Design review of the part built by this model. Coordinates are the model's own, in mm. A direction names the side the tool comes from. Coordinates: 2 decimals unless noted, no trailing zeros. Loops run counter-clockwise (first coordinate to the right, second up) from the corner with the lowest first, then second, coordinate; pieces in that order, holes last. Notation, with made-up numbers: M 27.25,-6 L 49.25,-6 A22 ccw 49.25,21 Z; hole C 76,1 d5. An arc over 180 degrees is marked long. Put each result on its own line as item: value. Start each with the question number.
(1) Clearance check with flat-ended pins moving along their axes: pin 1 (2 mm diameter, centred on y = 7, z = 7.5, fed in from -X); pin 2 (3.5 mm diameter, centred on x = 0, y = 9, fed in from -Z); pin 3 (3 mm diameter, centred on y = -2.5, z = 3.5, fed in from -X). State where each tip first meets the part, or that it passes through.
(2) Take a section at B-B, the plane x = 0. Count the separate pieces of the cut face and the enclosed holes in it, then the cut area to 4 significant figures.
(3) For faces 5 (the cylindrical face through (3.461, 9.056, 6.654)), 6 (the cylindrical face through (-7.493, -6.972, -0.33)), 7 (the conical face through (9.09, 0.17, -1.19)), list the 3-axis set-ups (+Z, -Z, +X, -X, +Y, -Y) from which the entire face can be reached by the end or side of a thin tool; tool diameter is ignored.
(4) Take a section at C-C, the plane y = 9. Give the boundary of the cut face in (x, z), then the cut area to 3 significant figures.
(5) Take a section at D-D, the plane y = -7.25. Give the boundary of the cut face in (x, z).
(6) The part is to be moulded in two halves that separate along X. For faces 1 (the cylindrical face through (11.547, 4.26, 4.788)), 2 (the cylindrical face through (-1.5, 9.07, 5.58)), 3 (the flat face through (0, 5, 8)), 4 (the cylindrical face through (-1.5, 9.07, -5.58)), say which applies: +X half, -X half, draft (parallel to the pull), parting line (faces both ways), or undercut.
(7) For probe 1 along X at (y, z) = (6.75, 0); probe 2 along Y at (x, z) = (0, -4.85); probe 3 along Y at (x, z) = (-6, 9.5), list the stretches that pass through material, from the lowest coordinate up. Write a range as [from, to].
(8) Take a section at A-A, the plane z = 0. Give the boundary of the cut face in (x, y).
```python
from build123d import *

# Parameters (mm, degrees)
SKETCH1_R                = 7.5
SKETCH1_R_2              = 4
BOSS_EXTRUDE1_DEPTH      = 13
BOSS_EXTRUDE1_DEPTH_BACK = 9
SKETCH1_4_R              = 12.5
SKETCH1_4_R_2            = 7.5
BOSS_EXTRUDE2_DEPTH      = 5
BOSS_EXTRUDE2_DEPTH_BACK = 5
SKETCH3_R                = 1.5
CUT_EXTRUDE1_DEPTH       = 13.5
CUT_EXTRUDE1_DEPTH_BACK  = 13.5


with BuildPart() as part:
    # Sketch1 → Boss-Extrude1 (new body, two sides)
    with BuildSketch(Plane(origin=(0, 0, 0), x_dir=(1, 0, 0), z_dir=(0, 1, 0))) as boss_extrude1_sk:
        Circle(SKETCH1_R)
        Circle(SKETCH1_R_2, mode=Mode.SUBTRACT)
    extrude(amount=BOSS_EXTRUDE1_DEPTH)
    extrude(boss_extrude1_sk.sketch, amount=-BOSS_EXTRUDE1_DEPTH_BACK)

    # Sketch1<4> → Boss-Extrude2 (add, two sides)
    with BuildSketch(Plane(origin=(0, 0, 0), x_dir=(1, 0, 0), z_dir=(0, 1, 0))) as boss_extrude2_sk:
        Circle(SKETCH1_4_R)
        Circle(SKETCH1_4_R_2, mode=Mode.SUBTRACT)
    extrude(amount=BOSS_EXTRUDE2_DEPTH)
    extrude(boss_extrude2_sk.sketch, amount=-BOSS_EXTRUDE2_DEPTH_BACK)

    # Sketch2 → Cut-Revolve1 (revolve, cut)
    with BuildSketch(Plane(origin=(0, 0, 0), x_dir=(0, 0, -1), z_dir=(1, 0, 0))):
        Polygon((-12.5, 3.5), (-9, 0), (-12.5, -3.5), align=None)
    revolve(axis=Axis((0, 0, 0), (0, 1, 0)), mode=Mode.SUBTRACT)

    # Sketch3 → Cut-Extrude1 (cut, two sides)
    with BuildSketch(Plane.XY) as cut_extrude1_sk:
        with Locations((0, 9)):
            Circle(SKETCH3_R)
    extrude(amount=CUT_EXTRUDE1_DEPTH, mode=Mode.SUBTRACT)
    extrude(cut_extrude1_sk.sketch, amount=-CUT_EXTRUDE1_DEPTH_BACK, mode=Mode.SUBTRACT)


solid = part.part
```
Computed values:
1. pin 1: stops at x = -3.74
1. pin 2: stops at z = -7.5
1. pin 3: stops at x = -12.27
2. separate pieces: 4
2. enclosed holes: 0
2. area: 208.5 mm^2
3. face 5: +Y
3. face 6: -Y
3. face 7: none
4. outline: M -1.5,-7.35 L -1.5,-3.71 A4 cw -1.5,3.71 L -1.5,7.35 A7.5 ccw Z; M 1.5,-7.35 A7.5 ccw 1.5,7.35 L 1.5,3.71 A4 cw 1.5,-3.71 Z
4. area: 105 mm^2
5. outline: C 0,0 d15; hole C 0,0 d8
6. face 1: parting line
6. face 2: undercut
6. face 3: draft
6. face 4: undercut
7. probe 1: x = [-7.5, -4], [4, 7.5]
7. probe 2: y = [-9, 7.5], [10.5, 13]
7. probe 3: y = [-5, -2.24], [2.24, 5]
8. outline: M -12.5,-5 L -7.5,-5 L -7.5,-9 L -4,-9 L -4,13 L -7.5,13 L -7.5,5 L -12.5,5 L -12.5,3.5 L -9,0 L -12.5,-3.5 Z; M 4,-9 L 7.5,-9 L 7.5,-5 L 12.5,-5 L 12.5,-3.5 L 9,0 L 12.5,3.5 L 12.5,5 L 7.5,5 L 7.5,13 L 4,13 Z
